Geometry: final body of the model. Coordinates: model frame, mm. Coordinates: 2 decimals unless noted, no trailing zeros. Loops run counter-clockwise (first coordinate to the right, second up) from the corner with the lowest first, then second, coordinate; pieces in that order, holes last. Notation, with made-up numbers: M -0.5,24.5 L 12.5,24.5 A19 cw 12.5,47.5 Z; hole C 55,-8.5 d9. An arc over 180 degrees is marked long. Write each question's results on one line, items separated by ' | '. Start each with the question number.
from build123d import *

# Parameters (mm, degrees)
CROQUIS1_R              = 5
SALIENTE_EXTRUIR1_DEPTH = 0.7
CORTAR_EXTRUIR1_REACH   = 2.7
REDONDEO1_R             = 1.1


with BuildPart() as part:
    # Croquis1 → Saliente-Extruir1 (new body)
    with BuildSketch(Plane.XY):
        Circle(CROQUIS1_R)
    extrude(amount=SALIENTE_EXTRUIR1_DEPTH)

    # Croquis2 → Cortar-Extruir1 (cut, up to next)
    with BuildSketch(Plane.XY.offset(0.7), mode=Mode.PRIVATE) as cortar_extruir1_sk1:
        with BuildLine():
            ThreePointArc((-0.598421585, 2.424539493), (0, 2.3), (0.598421585, 2.424539493))
            ThreePointArc((0.598421585, 2.424539493), (2.622160983, 1.904699976), (2.61328938, -0.184719936))
            ThreePointArc((2.61328938, -0.184719936), (1.528064828, -2.366548348), (1.4, -4.8))
            ThreePointArc((1.4, -4.8), (0, -5), (-1.4, -4.8))
            ThreePointArc((-1.4, -4.8), (-1.528064828, -2.366548348), (-2.61328938, -0.184719936))
            ThreePointArc((-2.61328938, -0.184719936), (-2.622160983, 1.904699976), (-0.598421585, 2.424539493))
        make_face()
    cortar_extruir1_tool1 = extrude(cortar_extruir1_sk1.sketch, amount=-CORTAR_EXTRUIR1_REACH, mode=Mode.PRIVATE) & part.part
    add(cortar_extruir1_tool1.solids().sort_by_distance((0, -0.660031, 0.7))[0], mode=Mode.SUBTRACT)

    # Redondeo1
    redondeo1_edges = [part.edges().sort_by_distance(p)[0] for p in [
        (1.4, -4.8, 0.35),
        (-1.4, -4.8, 0.35),
    ]]
    fillet(redondeo1_edges, radius=REDONDEO1_R)


solid = part.part
Item 1: Ray query, L1, parallel to X at y = -3, z = 0.35; L2, parallel to X at y = 2.25, z = 0.15; L3, parallel to X at y = 2.75, z = 0.2. Return the intervals inside material, ascending. Write a range as [from, to].
Item 2: Section B-B, the plane x = 0. Return loops of the section in (y, z), plus the area to 3 significant figures.
Item 3: Section A-A, the plane y = 0. Return loops of the section in (x, z), plus the area to 3 significant figures.
Item 4: Pull-direction query (Y, two-part tool) for faces 1 (the flat face through (0, 3, 0.7)), 2 (the cylindrical face through (0.171, 4.997, 0.345)), 3 (the cylindrical face through (-1.86, -1.43, 0.35)), 4 (the cylindrical face through (1.877, -1.391, 0.355)); classes: released by +Y, released by -Y, zero draft, split by the parting line, or undercut.
Item 5: Section C-C, the plane y = 1.5. Return loops of the section in (x, z), plus the area to 3 significant figures.
Item 6: Contact query for a flat-ended pin moving along its axis: P1, Ø3, axis at x = 0, y = 2, coming from the -Z side. Output: stop coordinate, or through.
Item 7: Section D-D, the plane y = 3. Return loops of the section in (x, z), plus the area to 3 significant figures.
Solutions:
1) L1: x = [-4, -1.42], [1.42, 4] | L2: x = [-4.47, -2.26], [2.26, 4.47] | L3: x = [-4.18, 4.18]
2) outline: M 2.3,0 L 5,0 L 5,0.7 L 2.3,0.7 Z | area: 1.89 mm²
3) outline: M -5,0 L -2.74,0 L -2.74,0.7 L -5,0.7 Z; M 2.74,0 L 5,0 L 5,0.7 L 2.74,0.7 Z | area: 3.16 mm²
4) face 1: zero draft | face 2: split by the parting line | face 3: undercut | face 4: undercut
5) outline: M -4.77,0 L -2.85,0 L -2.85,0.7 L -4.77,0.7 Z; M 2.85,0 L 4.77,0 L 4.77,0.7 L 2.85,0.7 Z | area: 2.68 mm²
6) P1: stops at z = 0
7) outline: M -4,0 L 4,0 L 4,0.7 L -4,0.7 Z | area: 5.60 mm²
